Read the model definition and answer for the solid it produces. Units are mm, in the model's axes. A direction names the side the tool comes from. Coordinates: 2 decimals unless noted, no trailing zeros. Order: outer loops, then holes, each group sorted by start corner. A loop starts at its lowest first (then second) coordinate and runs counter-clockwise, first axis right, second up. Notation, with made-up numbers: (-22, 47.25) -> (-4, 47.25) arc R22 cw to (-4, 79.25) -> close; hole circle Ø10 at (69, 21). An arc over 180 degrees is marked (long way). Answer in a Markdown table with one row per item.
from build123d import *

# Parameters (mm, degrees)
SKETCH1_W            = 27
SKETCH1_H            = 27
SKETCH1_W_2          = 23
SKETCH1_H_2          = 23
BOSS_EXTRUDE1_DEPTH  = 2
SKETCH2_W            = 27
SKETCH2_H            = 27
BOSS_EXTRUDE2_DEPTH  = 2
SKETCH12_W           = 8
SKETCH12_H           = 4
BOSS_EXTRUDE9_DEPTH  = 8
CIRPATTERN1_COUNT    = 4
SKETCH20_R           = 2
CUT_EXTRUDE11_DEPTH  = 4
CIRPATTERN2_COUNT    = 4
SKETCH13_R           = 1.75
CUT_EXTRUDE4_DEPTH   = 2
LPATTERN3_COUNT      = 6
LPATTERN3_PITCH      = 3.75
LPATTERN3_COUNT_DIR2 = 6
LPATTERN3_PITCH_DIR2 = 3.75
SKETCH14_W           = 27
SKETCH14_H           = 27
SKETCH14_W_2         = 23
SKETCH14_H_2         = 23
BOSS_EXTRUDE10_DEPTH = 8.5
BOSS_EXTRUDE11_DEPTH = 23
SKETCH18_W           = 27
SKETCH18_H           = 27
BOSS_EXTRUDE12_DEPTH = 2
SKETCH17_R           = 4.25
CUT_EXTRUDE10_DEPTH  = 2
SKETCH19_R           = 0.5
BOSS_EXTRUDE13_DEPTH = 6.51087


with BuildPart() as part:
    # Sketch1 → Boss-Extrude1 (new body)
    with BuildSketch(Plane(origin=(0, 0, 0), x_dir=(1, 0, 0), z_dir=(0, 1, 0))):
        Rectangle(SKETCH1_W, SKETCH1_H)
        Rectangle(SKETCH1_W_2, SKETCH1_H_2, mode=Mode.SUBTRACT)
    extrude(amount=BOSS_EXTRUDE1_DEPTH)

    # Sketch2 → Boss-Extrude2 (add)
    with BuildSketch(Plane.XZ):
        Rectangle(SKETCH2_W, SKETCH2_H)
    extrude(amount=BOSS_EXTRUDE2_DEPTH)

    # Sketch12 → Boss-Extrude9 (add)
    with BuildSketch(Plane.ZY.offset(13.5)):
        Rectangle(SKETCH12_W, SKETCH12_H)
    boss_extrude9 = extrude(amount=BOSS_EXTRUDE9_DEPTH)

    # CirPattern1: Boss-Extrude9 ×4 about axis
    cirpattern1_axis = Axis((0, 0, 0), (0, 1, 0))
    for i in range(1, CIRPATTERN1_COUNT):
        add(boss_extrude9.rotate(cirpattern1_axis, i * 360 / CIRPATTERN1_COUNT))

    # Sketch20 → Cut-Extrude11 (cut)
    with BuildSketch(Plane(origin=(0, 2, 0), x_dir=(1, 0, 0), z_dir=(0, 1, 0))):
        with Locations((0, -17.5)):
            Circle(SKETCH20_R)
    cut_extrude11 = extrude(amount=-CUT_EXTRUDE11_DEPTH, mode=Mode.SUBTRACT)

    # CirPattern2: Cut-Extrude11 ×4 about axis
    cirpattern2_axis = Axis((0, 0, 0), (0, 1, 0))
    for i in range(1, CIRPATTERN2_COUNT):
        add(cut_extrude11.rotate(cirpattern2_axis, i * 360 / CIRPATTERN2_COUNT), mode=Mode.SUBTRACT)

    # Sketch13 → Cut-Extrude4 (cut)
    with BuildSketch(Plane(origin=(0, 0, 0), x_dir=(1, 0, 0), z_dir=(0, 1, 0))):
        with Locations((9.5, 9.5)):
            Circle(SKETCH13_R)
    cut_extrude4 = extrude(amount=-CUT_EXTRUDE4_DEPTH, mode=Mode.SUBTRACT)

    # LPattern3: Cut-Extrude4 6 × 6
    with Locations(*[(-j * LPATTERN3_PITCH_DIR2, 0, i * LPATTERN3_PITCH) for i in range(LPATTERN3_COUNT) for j in range(LPATTERN3_COUNT_DIR2) if (i, j) != (0, 0)]):
        add(cut_extrude4, mode=Mode.SUBTRACT)

    # Sketch14 → Boss-Extrude10 (add)
    with BuildSketch(Plane.XZ.offset(2)):
        Rectangle(SKETCH14_W, SKETCH14_H)
        Rectangle(SKETCH14_W_2, SKETCH14_H_2, mode=Mode.SUBTRACT)
    extrude(amount=BOSS_EXTRUDE10_DEPTH)

    # Sketch16 → Boss-Extrude11 (add)
    with BuildSketch(Plane.ZY.offset(-11.5)):
        Polygon((11.5, -10.5), (-11.5, -10.5), (-11.5, -9.5), (11.5, -3), align=None)
    extrude(amount=BOSS_EXTRUDE11_DEPTH)

    # Sketch18 → Boss-Extrude12 (add)
    with BuildSketch(Plane.XZ.offset(10.5)):
        Rectangle(SKETCH18_W, SKETCH18_H)
    extrude(amount=BOSS_EXTRUDE12_DEPTH)

    # Sketch17 → Cut-Extrude10 (cut)
    with BuildSketch(Plane(origin=(0, 0, -13.5), x_dir=(-1, 0, 0), z_dir=(0, 0, -1))):
        with Locations((0, -6.25)):
            Circle(SKETCH17_R)
    extrude(amount=-CUT_EXTRUDE10_DEPTH, mode=Mode.SUBTRACT)

    # Sketch19 → Boss-Extrude13 (add)
    with BuildSketch(Plane.XZ.offset(2)):
        Circle(SKETCH19_R)
        with Locations((3.75, 0)):
            Circle(SKETCH19_R)
        with Locations((0, 3.75)):
            Circle(SKETCH19_R)
        with Locations((-3.75, 3.75)):
            Circle(SKETCH19_R)
        with Locations((3.75, 3.75)):
            Circle(SKETCH19_R)
        with Locations((7.5, 3.75)):
            Circle(SKETCH19_R)
        with Locations((7.5, 7.5)):
            Circle(SKETCH19_R)
        with Locations((3.75, 7.5)):
            Circle(SKETCH19_R)
        with Locations((0, 7.5)):
            Circle(SKETCH19_R)
        with Locations((-3.75, 7.5)):
            Circle(SKETCH19_R)
        with Locations((-7.5, 7.5)):
            Circle(SKETCH19_R)
        with Locations((-7.5, 3.75)):
            Circle(SKETCH19_R)
        with Locations((-7.5, 0)):
            Circle(SKETCH19_R)
        with Locations((-3.75, 0)):
            Circle(SKETCH19_R)
        with Locations((-3.75, -3.75)):
            Circle(SKETCH19_R)
        with Locations((-7.5, -3.75)):
            Circle(SKETCH19_R)
        with Locations((-7.5, -7.5)):
            Circle(SKETCH19_R)
        with Locations((-3.75, -7.5)):
            Circle(SKETCH19_R)
        with Locations((0, -7.5)):
            Circle(SKETCH19_R)
        with Locations((0, -3.75)):
            Circle(SKETCH19_R)
        with Locations((3.75, -3.75)):
            Circle(SKETCH19_R)
        with Locations((3.75, -7.5)):
            Circle(SKETCH19_R)
        with Locations((7.5, -7.5)):
            Circle(SKETCH19_R)
        with Locations((7.5, -3.75)):
            Circle(SKETCH19_R)
        with Locations((7.5, 0)):
            Circle(SKETCH19_R)
    extrude(amount=BOSS_EXTRUDE13_DEPTH)


solid = part.part
Q1. The part is cut by section A-A (x = 17.5). Write down the section's boundary in (y, z), then the cut area to 3 significant figures.
Outcome:
| item | result |
|---|---|
| outline | (-2, -4) -> (2, -4) -> (2, -2) -> (-2, -2) -> close; (-2, 2) -> (2, 2) -> (2, 4) -> (-2, 4) -> close |
| area | 16.0 mm² |
Q2. Consider line 1 (X direction, y = -5.5, z = -6.5); line 2 (X direction, y = -8.5, z = -12); line 3 (Y direction, x = -18.5, z = -2). Determine where each line is inside the solid, lowest interval first.
Outcome:
| item | result |
|---|---|
| line 1 | -13.5 to -11.5, 11.5 to 13.5 |
| line 2 | -13.5 to -3.61, 3.61 to 13.5 |
| line 3 | -2 to 2 |
Q3. The part is cut by section D-D (x = 12.5). Write down the section's boundary in (y, z).
Outcome:
| item | result |
|---|---|
| outline | (-12.5, -13.5) -> (2, -13.5) -> (2, 13.5) -> (-12.5, 13.5) -> close |
Q4. For faces 1 (the face through (-7.023, -4.701, -3.6)), 2 (the face through (0, 0, 21.5)), 3 (the face through (5.522, -0.986, -11.235)), determine the directions among +Z, -Z, +X, -X, +Y, -Y from which every point of the face is accessible in a straight line to the end or side of a thin tool.
Outcome:
| item | result |
|---|---|
| face 1 | none |
| face 2 | +Z, +X, -X, +Y, -Y |
| face 3 | +Y |
Q5. The part is cut by section B-B (x = -9.25). Give the number of separate pieces and of enclosed holes in the cut face, then the cut area to 3 significant figures.
Outcome:
| item | result |
|---|---|
| separate pieces | 6 |
| enclosed holes | 0 |
| area | 206 mm² |
Q6. For a pull along Y with two mould halves and no side action, classify faces 4 (the face through (-3.815, -4.701, -3.254)), 5 (the face through (5.37, -0.99, 7.21)), 6 (the face through (0, 0, 1)), 7 (the face through (0, -2, -1)) as pulls with the +Y half, pulls with the -Y half, needs draft (parallel to the pull), parting line crosses it, or undercut.
Outcome:
| item | result |
|---|---|
| face 4 | undercut |
| face 5 | needs draft |
| face 6 | pulls with the +Y half |
| face 7 | undercut |
Q7. The part is cut by section C-C (z = 14.5). Write down the section's boundary in (x, y), then the cut area to 3 significant figures.
Outcome:
| item | result |
|---|---|
| outline | (-4, -2) -> (4, -2) -> (4, 2) -> (-4, 2) -> close |
| area | 32.0 mm² |
Q8. Given pin 1 (4 mm diameter, centred on x = 5.75, z = 1.75, fed in from +Y); pin 2 (1.5 mm diameter, centred on x = -11.5, y = -1, fed in from -Z); pin 3 (6 mm diameter, centred on x = 13, y = -4, fed in from +Z), each flat-ended and moving along its own axis, determine where each tip first touches the part or whether it passes through.
Outcome:
| item | result |
|---|---|
| pin 1 | y = 0 |
| pin 2 | z = -13.5 |
| pin 3 | z = 13.5 |
